```python
from build123d import *

# Parameters (mm, degrees)
SKETCH1_R           = 3.175
BOSS_EXTRUDE1_DEPTH = 11.43
SKETCH2_R           = 9.776464607
CUT_EXTRUDE1_DEPTH  = 7.62


with BuildPart() as part:
    # Sketch1 → Boss-Extrude1 (new body)
    with BuildSketch(Plane(origin=(0, 0, 0), x_dir=(0, 0, -1), z_dir=(1, 0, 0))):
        with BuildLine():
            Line((6.35, 82.55), (-6.35, 82.55))
            Line((-6.35, 82.55), (-6.35, 63.181702256))
            ThreePointArc((-6.35, 63.181702256), (-44.901280605, 44.901280605), (-63.181702256, 6.35))
            Line((-63.181702256, 6.35), (-82.55, 6.35))
            Line((-82.55, 6.35), (-82.55, -6.35))
            Line((-82.55, -6.35), (-63.181702256, -6.35))
            ThreePointArc((-63.181702256, -6.35), (-44.901280605, -44.901280605), (-6.35, -63.181702256))
            Line((-6.35, -63.181702256), (-6.35, -82.55))
            Line((-6.35, -82.55), (6.35, -82.55))
            Line((6.35, -82.55), (6.35, -63.181702256))
            ThreePointArc((6.35, -63.181702256), (44.901280605, -44.901280605), (63.181702256, -6.35))
            Line((63.181702256, -6.35), (82.55, -6.35))
            Line((82.55, -6.35), (82.55, 6.35))
            Line((82.55, 6.35), (63.181702256, 6.35))
            ThreePointArc((63.181702256, 6.35), (44.901280605, 44.901280605), (6.35, 63.181702256))
            Line((6.35, 63.181702256), (6.35, 82.55))
        make_face()
        Circle(SKETCH1_R, mode=Mode.SUBTRACT)
    extrude(amount=BOSS_EXTRUDE1_DEPTH)

    # Sketch2 → Cut-Extrude1 (cut)
    with BuildSketch(Plane.ZY):
        Circle(SKETCH2_R)
    extrude(amount=-CUT_EXTRUDE1_DEPTH, mode=Mode.SUBTRACT)


solid = part.part
```
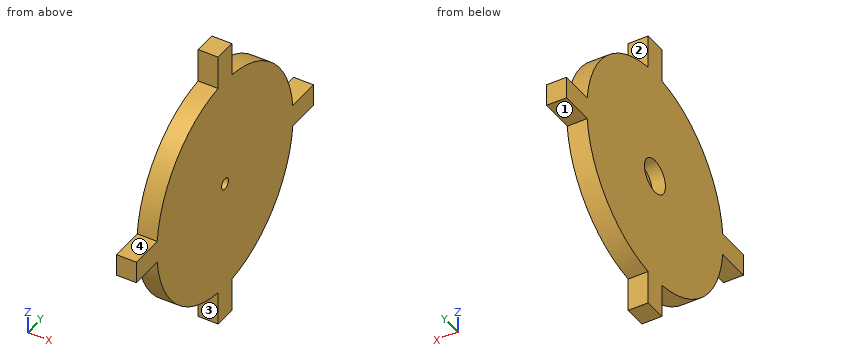
CAD build for the part. Positions are in the model's coordinates, mm. Face numbers are marked on the shaded views. A direction names the side the tool comes from. Round coordinates to 2 decimals unless told otherwise and drop trailing zeros. Write each loop counter-clockwise with the first axis right and the second up, starting at its lowest first coordinate (ties: lowest second). Pieces come first, ordered by that corner, then holes. Notation, with made-up numbers: M 56,3.25 L 109,3.25 A25 cw 109,23.25 Z; hole C 66.5,82.25 d3. An arc over 180 degrees is marked long. One line per question, with ' | ' between items.
1. Cut at A-A on z = 0. Write the cut outline in (x, y) (3 decimals).
Working result:
outline: M 0,-82.55 L 11.43,-82.55 L 11.43,-3.175 L 7.62,-3.175 L 7.62,-9.776 L 0,-9.776 Z; M 0,9.776 L 7.62,9.776 L 7.62,3.175 L 11.43,3.175 L 11.43,82.55 L 0,82.55 Z
2. Probe L1, parallel to Y at x = 3, z = 0; L2, parallel to Z at x = 5.25, y = 0.5; L3, parallel to Z at x = 9.4, y = 0 (3 decimals). List the from-to ranges inside material, lowest first. Write a range as from..to.
Working result:
L1: -82.55..-9.78, 9.78..82.55 | L2: -82.55..-9.76, 9.76..82.55 | L3: -82.55..-3.175, 3.175..82.55
3. Pin check, flat tips, straight feed: pin 1 Ø10 at (y, z) = (0, 0) entering from -X; pin 2 Ø3.5 at (x, y) = (4.5, -70.5) entering from +Z; pin 3 Ø2 at (x, y) = (1.5, 24.5) entering from -Z; pin 4 Ø5 at (x, z) = (8, -7) entering from +Y. Stop position of each tip, or through.
Working result:
pin 1: x = 7.62 | pin 2: z = 6.35 | pin 3: z = -58.99 | pin 4: y = 82.55
4. Cut at C-C on x = 5.25. Write the cut outline in (y, z), and give its area (3 significant figures).
Working result:
outline: M -82.55,-6.35 L -63.18,-6.35 A63.5 ccw -6.35,-63.18 L -6.35,-82.55 L 6.35,-82.55 L 6.35,-63.18 A63.5 ccw 63.18,-6.35 L 82.55,-6.35 L 82.55,6.35 L 63.18,6.35 A63.5 ccw 6.35,63.18 L 6.35,82.55 L -6.35,82.55 L -6.35,63.18 A63.5 ccw -63.18,6.35 L -82.55,6.35 Z; hole C 0,0 d19.55 | area: 13,300 mm2
5. Which spindle directions (+Z, -Z, +X, -X, +Y, -Y) get a long thin tool onto all of the face, cutting with end or side? Do the marked faces 1, 2, 3 and 4. Say none if no direction does.
Working result:
face 1: -Z, +X, -X, +Y | face 2: +Z, +X, -X, +Y | face 3: -Z, +X, -X, -Y | face 4: +Z, +X, -X, -Y
6. Cut at D-D on z = 69. Write the cut outline in (x, y), and give its area (3 significant figures).
Working result:
outline: M 0,-6.35 L 11.43,-6.35 L 11.43,6.35 L 0,6.35 Z | area: 145 mm2
